Input: part model. Units: mm. Frame: model coordinates. A direction names the side the tool comes from. Round coordinates to 2 decimals unless told otherwise and drop trailing zeros. Write each loop counter-clockwise with the first axis right and the second up, starting at its lowest first coordinate (ties: lowest second). Pieces come first, ordered by that corner, then holes. Notation, with made-up numbers: (40, -26.5) - (76, -26.5) arc R7 ccw to (76, -14.5) - close; hole circle Ø5 at (46.25, -4.75). An arc over 180 degrees is marked (long way). Use one line per item in the form item = value.
```python
from build123d import *

# Parameters (mm, degrees)
SKETCH1_W                      = 103.175
SKETCH1_H                      = 103.175
SKETCH1_W_2                    = 100
SKETCH1_H_2                    = 100
BULKSHELLEXTRUDE_DEPTH         = 376.8
SKETCH14_W                     = 77.775
SKETCH14_H                     = 351.4
SIDEWALLCUT_DEPTH              = 103.1875
SIDEWALLCUTPATTERN_COUNT       = 4
SKETCH20_W                     = 77.775
SKETCH20_H                     = 12.7
CENTERSUPPORT_DEPTH            = 1.5875
CENTERSUPPORTPATTERNCIRC_COUNT = 4
SKETCH22_W                     = 100
SKETCH22_H                     = 376.8
CUT_EXTRUDE4_DEPTH             = 103.1875
SKETCH23_W                     = 1.5875
SKETCH23_H                     = 376.8
BOSS_EXTRUDE1_DEPTH            = 1.5875
SKETCH24_W                     = 1.5875
SKETCH24_H                     = 376.8
BOSS_EXTRUDE2_DEPTH            = 12.7


with BuildPart() as part:
    # Sketch1 → BulkShellExtrude (new body)
    with BuildSketch(Plane(origin=(0, 0, 0), x_dir=(1, 0, 0), z_dir=(0, 1, 0))):
        Rectangle(SKETCH1_W, SKETCH1_H)
        Rectangle(SKETCH1_W_2, SKETCH1_H_2, mode=Mode.SUBTRACT)
    extrude(amount=BULKSHELLEXTRUDE_DEPTH)

    # Sketch14 → SideWallCut (cut)
    with BuildSketch(Plane(origin=(51.5875, 0, 0), x_dir=(0, 0, -1), z_dir=(1, 0, 0))):
        with Locations((0, 188.4)):
            Rectangle(SKETCH14_W, SKETCH14_H)
    sidewallcut = extrude(amount=-SIDEWALLCUT_DEPTH, mode=Mode.SUBTRACT)

    # SideWallCutPattern: SideWallCut ×4 about axis
    sidewallcutpattern_axis = Axis((0, 0, 0), (0, 1, 0))
    for i in range(1, SIDEWALLCUTPATTERN_COUNT):
        add(sidewallcut.rotate(sidewallcutpattern_axis, i * 360 / SIDEWALLCUTPATTERN_COUNT), mode=Mode.SUBTRACT)

    # Sketch20 → CenterSupport (add)
    with BuildSketch(Plane.XY.offset(51.5875)):
        with Locations((0, 188.4)):
            Rectangle(SKETCH20_W, SKETCH20_H)
    centersupport = extrude(amount=-CENTERSUPPORT_DEPTH)

    # CenterSupportPatternCirc: CenterSupport ×4 about axis
    centersupportpatterncirc_axis = Axis((0, 0, 0), (0, 1, 0))
    for i in range(1, CENTERSUPPORTPATTERNCIRC_COUNT):
        add(centersupport.rotate(centersupportpatterncirc_axis, i * 360 / CENTERSUPPORTPATTERNCIRC_COUNT))

    # Sketch22 → Cut-Extrude4 (cut)
    with BuildSketch(Plane(origin=(51.5875, 0, 0), x_dir=(0, 0, -1), z_dir=(1, 0, 0))):
        with Locations((0, 188.4)):
            Rectangle(SKETCH22_W, SKETCH22_H)
    extrude(amount=-CUT_EXTRUDE4_DEPTH, mode=Mode.SUBTRACT)


with BuildPart() as body_2:
    # of the pieces the cut leaves, the one that is kept (cut_extrude4_keep)
    add(part.part.solids().sort_by_distance((51.5875, 0, 51.5875))[0])

    # Sketch23 → Boss-Extrude1 (add)
    with BuildSketch(Plane(origin=(51.5875, 0, 0), x_dir=(0, 0, -1), z_dir=(1, 0, 0))):
        with Locations((-50.79375, 188.4)):
            Rectangle(SKETCH23_W, SKETCH23_H)
    boss_extrude1 = extrude(amount=BOSS_EXTRUDE1_DEPTH)

    # Mirror1: Boss-Extrude1 across plane
    add(boss_extrude1.mirror(Plane(origin=(0, 0, 0), x_dir=(0, 0, 1), z_dir=(1, 0, 0))))

    # Sketch24 → Boss-Extrude2 (add)
    with BuildSketch(Plane(origin=(0, 0, 50), x_dir=(-1, 0, 0), z_dir=(0, 0, -1))):
        with Locations((-52.38125, 188.4)):
            Rectangle(SKETCH24_W, SKETCH24_H)
        with Locations((52.38125, 188.4)):
            Rectangle(SKETCH24_W, SKETCH24_H)
    extrude(amount=BOSS_EXTRUDE2_DEPTH)


solid = body_2.part
```
(1) Cut plane A-A on x = 28. Output: boundary loops of the cut face in (y, z), then the cut area to 3 significant figures.
Derived:
outline = (0, 50) - (12.7, 50) - (12.7, 51.59) - (0, 51.59) - close; (182.05, 50) - (194.75, 50) - (194.75, 51.59) - (182.05, 51.59) - close; (364.1, 50) - (376.8, 50) - (376.8, 51.59) - (364.1, 51.59) - close
area = 60.5 mm^2
(2) Material intervals for L1, parallel to X at y = 345.5, z = 43 (1 decimal); L2, parallel to X at y = 112.5, z = 51 (1 decimal); L3, parallel to Z at x = -47.5, y = 37.5, sorted ascending.
Derived:
L1 = -53.2 to -51.6, 51.6 to 53.2
L2 = -53.2 to -38.9, 38.9 to 53.2
L3 = 50 to 51.59
(3) Access query for faces 1 (the face through (4, 188, 51.588)), 2 (the face through (-51.588, 186, 44)). Directions: +Z, -Z, +X, -X, +Y, -Y. A direction counts if a zero-diameter tool reaches every point of the face in a straight line with its end or side. Return the directions, or none.
Derived:
face_1 = +Z, +X, -X, +Y, -Y
face_2 = -Z, +Y, -Y
(4) Cut plane B-B on y = 214. Output: boundary loops of the cut face in (x, z) (1 decimal).
Derived:
outline = (-53.2, 37.3) - (-51.6, 37.3) - (-51.6, 50) - (-38.9, 50) - (-38.9, 51.6) - (-53.2, 51.6) - close; (38.9, 50) - (51.6, 50) - (51.6, 37.3) - (53.2, 37.3) - (53.2, 51.6) - (38.9, 51.6) - close
(5) Cut plane C-C on z = 45.5. Output: boundary loops of the cut face in (x, y) (1 decimal).
Derived:
outline = (-53.2, 0) - (-51.6, 0) - (-51.6, 376.8) - (-53.2, 376.8) - close; (51.6, 0) - (53.2, 0) - (53.2, 376.8) - (51.6, 376.8) - close
(6) Draft query along X for faces 3 (the face through (51.588, 186, 44)), 4 (the face through (-53.175, 191, 45)), 5 (the face through (53.175, 186, 45)). Return one class per face: released by +X, released by -X, zero draft, split by the parting line, or undercut.
Derived:
face_3 = undercut
face_4 = released by -X
face_5 = released by +X
